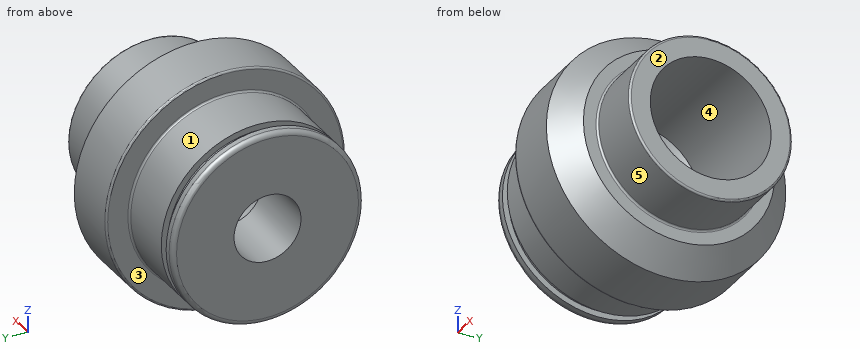
```python
from build123d import *


with BuildPart() as part:
    # Sketch1 → Base-Revolve (revolve)
    with BuildSketch(Plane.XY):
        with BuildLine():
            Line((0, 12.625), (0, 16.6))
            ThreePointArc((0, 16.6), (-0.117157288, 16.882842712), (-0.4, 17))
            Line((-0.4, 17), (-11.6, 17))
            ThreePointArc((-11.6, 17), (-11.882842712, 17.117157288), (-12, 17.4))
            Line((-12, 17.4), (-12, 20))
            Line((-12, 20), (-17, 25))
            Line((-17, 25), (-28.6, 25))
            ThreePointArc((-28.6, 25), (-28.882842712, 24.882842712), (-29, 24.6))
            Line((-29, 24.6), (-29, 20.4))
            ThreePointArc((-29, 20.4), (-29.117157288, 20.117157288), (-29.4, 20))
            Line((-29.4, 20), (-41, 20))
            Line((-41, 20), (-41, 18.75))
            Line((-41, 18.75), (-42.85, 18.75))
            Line((-42.85, 18.75), (-42.85, 20))
            Line((-42.85, 20), (-44, 20))
            ThreePointArc((-44, 20), (-44.707106781, 19.707106781), (-45, 19))
            Line((-45, 19), (-45, 7))
            Line((-45, 7), (-30.247595264, 7))
            Line((-30.247595264, 7), (-27, 12.625))
            Line((-27, 12.625), (0, 12.625))
        make_face()
    revolve(axis=Axis((0, 0, 0), (-1, 0, 0)))


solid = part.part
```
Can you work these out from the model? Positions are in its coordinate system, mm. Face numbers are marked on the shaded views. A direction names the side the tool comes from. Coordinates: 2 decimals unless noted, no trailing zeros. Order: outer loops, then holes, each group sorted by start corner. A loop starts at its lowest first (then second) coordinate and runs counter-clockwise, first axis right, second up. Notation, with made-up numbers: (56.5, 29.25) -> (106.5, 29.25) arc R33 ccw to (106.5, 58.25) -> close; hole circle Ø10 at (55, 38.5). An arc over 180 degrees is marked (long way). Write each question's results on one line, items separated by ' | '.
Item 1: If we mould it in two halves opening along Y, with no side actions, what happens to the marked faces 3, 4 and 5? For each: +Y half, -Y half, draft (parallel to the pull), parting line (faces both ways), or undercut.
Results are:
face 3: draft | face 4: undercut | face 5: parting line
Item 2: If I drill on line 1 along Z through (x, y) = (-19, 0) (3 decimals); line 2 along Y through (x, z) = (-34, 0); line 3 along Z through (x, y) = (-10, 0) (3 decimals), over which ranges is the centre line in solid material (lowest first)?
Results are:
line 1: -25 to -12.625, 12.625 to 25 | line 2: -20 to -7, 7 to 20 | line 3: -17 to -12.625, 12.625 to 17
Item 3: I want a section at A-A, the plane x = -24.5. Write out the boundary of the cut face in (y, z) (3 decimals), then the cut area to 3 significant figures.
Results are:
outline: circle Ø50 at (0, 0); hole circle Ø25.25 at (0, 0) | area: 1,460 mm²
Item 4: I want a section at B-B, the plane x = -40. Write out the boundary of the cut face in (y, z).
Results are:
outline: circle Ø40 at (0, 0); hole circle Ø14 at (0, 0)
Item 5: Which directions (+Z, -Z, +X, -X, +Y, -Y) give clear straight access to the entire face, cutting with the end or side of a thin tool? Please do the marked faces 1 and 2.
Results are:
face 1: -X | face 2: +Z, -Z, +X, +Y, -Y
Item 6: I'm going to push flat-ended pins straight in: pin 1 Ø20 at (y, z) = (6.5, -3.5) entering from +X; pin 2 Ø2 at (x, y) = (-35.5, -5) entering from +Z; pin 3 Ø4 at (x, z) = (-37, 1) entering from -Y; pin 4 Ø6 at (x, z) = (-12, -10) entering from +Y. Where does each tip first touch, or does it pass through?
Results are:
pin 1: x = 0 | pin 2: z = 19.6 | pin 3: y = -20 | pin 4: y = 20.98
